Read the model definition and answer for the solid it produces. Units are mm, in the model's axes. A direction names the side the tool comes from. Coordinates: 2 decimals unless noted, no trailing zeros. Write each loop counter-clockwise with the first axis right and the second up, starting at its lowest first coordinate (ties: lowest second). Pieces come first, ordered by that corner, then holes. Notation, with made-up numbers: M 62,-34.5 L 88,-34.5 A26 ccw 88,3.5 Z; hole C 4,39.5 d7. An arc over 180 degrees is marked long. Write item = value, one per line.
from build123d import *

# Parameters (mm, degrees)
F0_W        = 8
F0_H        = 5
F1_DEPTH    = 45
F0_R        = 2.5
F2_DEPTH    = 5
F3_DEPTH    = 10
F4_DEPTH    = 2
F5_T1_DEPTH = 5
F5_T3_DEPTH = 30
F5_T5_DEPTH = 33


# Not quite as in the source:
# - a fillet or chamfer that OpenCascade refuses, or shapes differently, is made with other operations: its cross-section is extruded or revolved along the edge and cut away or added


with BuildPart() as f1:
    # F0 (on Top) → F1 (new body)
    with BuildSketch(Plane.XY):
        with Locations((-5, -21)):
            Rectangle(F0_W, F0_H)
    extrude(amount=F1_DEPTH)

    # F0 (on Top) → F2 (join)
    with BuildSketch(Plane.XY):
        Polygon((9, 18.5), (-9, 18.5), (-9, -18.5), (-1, -18.5), (-1, 8.5), (9, 8.5), align=None)
        Polygon((1.6027649533, 9.4804546863), (-0.6796458767, 13.5662937924), (1.71758917, 17.5858391061), (6.3972350467, 17.5195453137), (8.6796458767, 13.4337062076), (6.28241083, 9.4141608939), align=None, mode=Mode.SUBTRACT)
        Polygon((1.71758917, 17.5858391061), (-0.6796458767, 13.5662937924), (1.6027649533, 9.4804546863), (6.28241083, 9.4141608939), (8.6796458767, 13.4337062076), (6.3972350467, 17.5195453137), align=None)
        with Locations((4, 13.5)):
            Circle(F0_R, mode=Mode.SUBTRACT)
    extrude(amount=F2_DEPTH)

    # F0 (on Top) → F3 (cut)
    with BuildSketch(Plane.XY):
        Polygon((1.71758917, 17.5858391061), (-0.6796458767, 13.5662937924), (1.6027649533, 9.4804546863), (6.28241083, 9.4141608939), (8.6796458767, 13.4337062076), (6.3972350467, 17.5195453137), align=None)
        with Locations((4, 13.5)):
            Circle(F0_R, mode=Mode.SUBTRACT)
    extrude(amount=F3_DEPTH, mode=Mode.SUBTRACT)

    # F0 (on Top) → F4 (join)
    with BuildSketch(Plane.XY):
        Polygon((1.71758917, 17.5858391061), (-0.6796458767, 13.5662937924), (1.6027649533, 9.4804546863), (6.28241083, 9.4141608939), (8.6796458767, 13.4337062076), (6.3972350467, 17.5195453137), align=None)
        with Locations((4, 13.5)):
            Circle(F0_R, mode=Mode.SUBTRACT)
    extrude(amount=F4_DEPTH)

    # F5: fillet of radius 5 on 7 edges, made by hand

    # F5_s2 → F5_t1 (join)
    with BuildSketch(Plane.XY):
        with BuildLine():
            ThreePointArc((-1, 3.5), (0.4644660941, 7.0355339059), (4, 8.5))
            Line((4, 8.5), (-1, 8.5))
            Line((-1, 8.5), (-1, 3.5))
        make_face()
    extrude(amount=F5_T1_DEPTH)

    # F5_s4 → F5_t3 (cut)
    with BuildSketch(Plane.XY.offset(-12.5)):
        with BuildLine():
            ThreePointArc((-9, 13.5), (-7.5355339059, 17.0355339059), (-4, 18.5))
            Line((-4, 18.5), (-9, 18.5))
            Line((-9, 18.5), (-9, 13.5))
        make_face()
        with BuildLine():
            ThreePointArc((4, 18.5), (7.5355339059, 17.0355339059), (9, 13.5))
            Line((9, 13.5), (9, 18.5))
            Line((9, 18.5), (4, 18.5))
        make_face()
        with BuildLine():
            ThreePointArc((9, 13.5), (7.5355339059, 9.9644660941), (4, 8.5))
            Line((4, 8.5), (9, 8.5))
            Line((9, 8.5), (9, 13.5))
        make_face()
    extrude(amount=F5_T3_DEPTH, mode=Mode.SUBTRACT)

    # F5_s6 → F5_t5 (cut)
    with BuildSketch(Plane.YZ.offset(-21.5)):
        with BuildLine():
            ThreePointArc((-23.5, 5), (-22.0355339059, 1.4644660941), (-18.5, 0))
            Line((-18.5, 0), (-23.5, 0))
            Line((-23.5, 0), (-23.5, 5))
        make_face()
        with BuildLine():
            ThreePointArc((-18.5, 45), (-22.0355339059, 43.5355339059), (-23.5, 40))
            Line((-23.5, 40), (-23.5, 45))
            Line((-23.5, 45), (-18.5, 45))
        make_face()
        with BuildLine():
            ThreePointArc((-18.5, 40), (-19.9644660941, 43.5355339059), (-23.5, 45))
            Line((-23.5, 45), (-18.5, 45))
            Line((-18.5, 45), (-18.5, 40))
        make_face()
    extrude(amount=F5_T5_DEPTH, mode=Mode.SUBTRACT)


solid = f1.part
Item 1: Flat-ended cylindrical pins translate along their axes: pin 1 (4 mm diameter, centred on x = 5.5, y = 13, fed in from +Z); pin 2 (4 mm diameter, centred on x = -6.5, z = 17, fed in from +Y). Find the tip coordinate at first contact, or state that the pin passes through.
Worked answers:
pin_1 = 2
pin_2 = -18.5
Item 2: For a pull along X with two mould halves and no side action, classify faces 1 (the face through (-5.06, -22.07, 1.5)), 2 (the face through (3.46, 11.06, 0.99)), 3 (the face through (-9, -19, 15)) as released by +X, released by -X, zero draft, split by the parting line, or undercut.
Worked answers:
face_1 = zero draft
face_2 = undercut
face_3 = released by -X
Item 3: Which of the six approach directions +Z, -Z, +X, -X, +Y, -Y give full straight-line access (tool end or side, diameter ignored) to faces 4 (the face through (-1, -19, 15)), 5 (the face through (0, 18.5, 2)), 6 (the face through (-4, 0, 5)), 7 (the face through (0.446, 11.552, 3.479)), 8 (the face through (-5.056, -22.812, 42.532))?
Worked answers:
face_4 = +Z, -Z, +X, -Y
face_5 = +Z, -Z, +X, -X, +Y
face_6 = +Z, +X, -X, +Y
face_7 = +Z
face_8 = +Z, +X, -X, -Y
Item 4: Consider line 1 along Y through (x, z) = (4, 1.25); line 2 along Y through (x, z) = (-1.5, 35.5); line 3 along Z through (x, y) = (-1.5, 3). Determine where each line is inside the solid, lowest interval first. Write a range as from..to.
Worked answers:
line_1 = 8.5..11, 16..18.5
line_2 = -23.5..-18.5
line_3 = 0..5
Item 5: Find section B-B (y = -1.5). Determine the outline of the cut face in (x, z), and give its area (3 significant figures).
Worked answers:
outline = M -9,0 L -1,0 L -1,5 L -9,5 Z
area = 40.0 mm²
Item 6: Find section C-C (z = 29.5). Determine the outline of the cut face in (x, y), and give its area (3 significant figures).
Worked answers:
outline = M -9,-23.5 L -1,-23.5 L -1,-18.5 L -9,-18.5 Z
area = 40.0 mm²
Item 7: Find section A-A (x = 2.5). Determine the outline of the cut face in (y, z).
Worked answers:
outline = M 8.27,0 L 11.5,0 L 11.5,2 L 9.47,2 L 9.47,5 L 8.27,5 Z; M 15.5,0 L 18.5,0 L 18.5,5 L 17.57,5 L 17.57,2 L 15.5,2 Z
